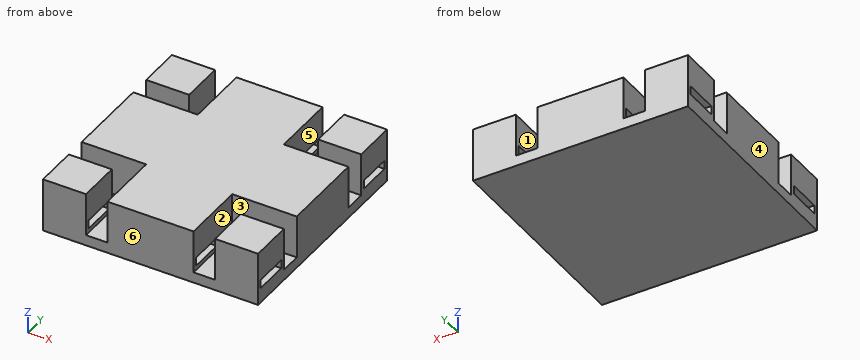
from build123d import *

# Parameters (mm, degrees)
F0_W     = 100
F0_H     = 100
F1_DEPTH = 100
F2_DEPTH = 25
F3_W     = 80
F3_H     = 20
F4_DEPTH = 5000


with BuildPart() as f1:
    # F0 (on Top) → F1 (new body)
    with BuildSketch(Plane.XY):
        Polygon((100, 100), (100, 250), (-100, 250), (-100, 100), (-250, 100), (-250, -100), (-100, -100), (-100, -250), (100, -250), (100, -100), (250, -100), (250, 100), align=None)
        with Locations((-200, -200)):
            Rectangle(F0_W, F0_H)
        with Locations((200, -200)):
            Rectangle(F0_W, F0_H)
        with Locations((200, 200)):
            Rectangle(F0_W, F0_H)
        with Locations((-200, 200)):
            Rectangle(F0_W, F0_H)
    extrude(amount=F1_DEPTH)

    # F0 (on Top) → F2 (join)
    with BuildSketch(Plane.XY):
        with Locations((200, -200)):
            Rectangle(F0_W, F0_H)
        Polygon((250, -150), (250, -100), (100, -100), (100, -250), (150, -250), (150, -150), align=None)
        Polygon((150, 150), (150, 250), (100, 250), (100, 100), (250, 100), (250, 150), align=None)
        with Locations((200, 200)):
            Rectangle(F0_W, F0_H)
        Polygon((100, 100), (100, 250), (-100, 250), (-100, 100), (-250, 100), (-250, -100), (-100, -100), (-100, -250), (100, -250), (100, -100), (250, -100), (250, 100), align=None)
        Polygon((-100, -100), (-250, -100), (-250, -150), (-150, -150), (-150, -250), (-100, -250), align=None)
        with Locations((-200, -200)):
            Rectangle(F0_W, F0_H)
        Polygon((-100, 100), (-100, 250), (-150, 250), (-150, 150), (-250, 150), (-250, 100), align=None)
        with Locations((-200, 200)):
            Rectangle(F0_W, F0_H)
    extrude(amount=-F2_DEPTH)

    # F3 (on face) → F4 (cut)
    with BuildSketch(Plane.YZ.offset(250)):
        with Locations((-200, 20)):
            Rectangle(F3_W, F3_H)
        with Locations((200, 20)):
            Rectangle(F3_W, F3_H)
    extrude(amount=-F4_DEPTH, mode=Mode.SUBTRACT)


solid = f1.part
Check sheet for the modelled part. Datum: model origin and axes. Units: mm. Face numbers are marked on the shaded views. A direction names the side the tool comes from. Give positions to 0.01 mm unless a question says otherwise; leave off trailing zeros. Write each loop counter-clockwise with the first axis right and the second up, starting at its lowest first coordinate (ties: lowest second). Pieces come first, ordered by that corner, then holes. Notation, with made-up numbers: (64.25, -29.5) -> (69.25, -29.5) arc R14 cw to (69.25, -20.5) -> close; hole circle Ø6 at (82.5, 18). An arc over 180 degrees is marked (long way). One line per item, written item: value. Start each with the question number.
Item 1: Section check C-C on z = 64.5. Record the cut outline in (x, y), then the cut area to 3 significant figures.
Item 2: Gauge pin test, flat ends, axial feed: pin 1 (12 mm diameter, centred on y = 174, z = 14.5, fed in from -X); pin 2 (8 mm diameter, centred on y = 127.5, z = 81, fed in from +X). Record the tip position at first contact, or that the pin passes through.
Item 3: Tool access check on the marked faces 1, 2 and 3. Record the directions out of +Z, -Z, +X, -X, +Y, -Y that give a thin tool (end or side, any length) a straight path to the whole face; none if there is none.
Item 4: Section check B-B on x = -12.5. Record the cut outline in (y, z), then the cut area to 3 significant figures.
Item 5: Material ranges on probe 1 along Y at (x, z) = (178, 79.5); probe 2 along Z at (x, y) = (76.5, -164), recorded low to high. Write a range as from..to.
Item 6: Section check A-A on y = 190.5. Record the cut outline in (x, z), then the cut area to 3 significant figures.
Item 7: Section check D-D on y = 133.5. Record the cut outline in (x, z).
Item 8: Draft check along X on the marked faces 4, 5 and 6. Enter one of: +X half, -X half, draft (parallel to the pull), parting line (faces both ways), or undercut.
Results list:
1. outline: (-250, -250) -> (-150, -250) -> (-150, -150) -> (-250, -150) -> close; (-250, -100) -> (-100, -100) -> (-100, -250) -> (100, -250) -> (100, -100) -> (250, -100) -> (250, 100) -> (100, 100) -> (100, 250) -> (-100, 250) -> (-100, 100) -> (-250, 100) -> close; (-250, 150) -> (-150, 150) -> (-150, 250) -> (-250, 250) -> close; (150, -250) -> (250, -250) -> (250, -150) -> (150, -150) -> close; (150, 150) -> (250, 150) -> (250, 250) -> (150, 250) -> close
1. area: 200,000 mm²
2. pin 1: x = -250
2. pin 2: x = 100
3. face 1: +Z, +Y
3. face 2: +Z, -Y
3. face 3: +Z, +X
4. outline: (-250, -25) -> (250, -25) -> (250, 100) -> (-250, 100) -> close; hole (-240, 10) -> (-160, 10) -> (-160, 30) -> (-240, 30) -> close; hole (160, 10) -> (240, 10) -> (240, 30) -> (160, 30) -> close
4. area: 59,300 mm²
5. probe 1: -250..-150, -100..100, 150..250
5. probe 2: -25..10, 30..100
6. outline: (-250, -25) -> (250, -25) -> (250, 10) -> (150, 10) -> (150, 0) -> (100, 0) -> (100, 10) -> (-100, 10) -> (-100, 0) -> (-150, 0) -> (-150, 10) -> (-250, 10) -> close; (-250, 30) -> (-150, 30) -> (-150, 100) -> (-250, 100) -> close; (-100, 30) -> (100, 30) -> (100, 100) -> (-100, 100) -> close; (150, 30) -> (250, 30) -> (250, 100) -> (150, 100) -> close
6. area: 44,500 mm²
7. outline: (-250, -25) -> (250, -25) -> (250, 0) -> (100, 0) -> (100, 100) -> (-100, 100) -> (-100, 0) -> (-250, 0) -> close
8. face 4: -X half
8. face 5: undercut
8. face 6: draft
